from build123d import *

# Parameters (mm, degrees)
BOX042_W                  = 13
BOX042_H                  = 42
BOX042_DEPTH              = 6
BOX043_W                  = 9
BOX043_H                  = 58
BOX043_DEPTH              = 2
CYLINDER024_R             = 20.5
CYLINDER024_DEPTH         = 23.5
FUSION001_PITCH_ANGLE     = -90
FUSION001_PLACEMENT_ANGLE = 90


with BuildPart() as cube022:
    # Box042 → Box042 (new body)
    with BuildSketch(Plane(origin=(-6.5, -21, 0), x_dir=(1, 0, 0), z_dir=(0, 0, 1))):
        with Locations((6.5, 21)):
            Rectangle(BOX042_W, BOX042_H)
    extrude(amount=BOX042_DEPTH)


with BuildPart() as cube023:
    # Box043 → Box043 (new body)
    with BuildSketch(Plane(origin=(-4.5, -29, 5.5), x_dir=(1, 0, 0), z_dir=(0, 0, 1))):
        with Locations((4.5, 29)):
            Rectangle(BOX043_W, BOX043_H)
    extrude(amount=BOX043_DEPTH)


with BuildPart() as speaker:
    # Cylinder024 → Cylinder024 (new body)
    with BuildSketch(Plane.XY):
        Circle(CYLINDER024_R)
    extrude(amount=CYLINDER024_DEPTH)

    # Fusion001: union Cube022, Cube023
    add(cube022.part)
    add(cube023.part)


with BuildPart() as speaker_1:
    # Fusion001 pitch: moved
    add(speaker.part.rotate(Axis((0, 0, 0), (0, 1, 0)), FUSION001_PITCH_ANGLE))


with BuildPart() as speaker_2:
    # Fusion001 placement: moved
    add(speaker_1.part.moved(Location((45, 86, 45))).rotate(Axis((45, 86, 45), (0, 0, 1)), FUSION001_PLACEMENT_ANGLE))


solid = speaker_2.part
Geometry: final body of the model. Coordinates: model frame, mm. A direction names the side the tool comes from. Round coordinates to 2 decimals unless told otherwise and drop trailing zeros. Write each loop counter-clockwise with the first axis right and the second up, starting at its lowest first coordinate (ties: lowest second). Pieces come first, ordered by that corner, then holes. Notation, with made-up numbers: M 84,-22 L 130,-22 A10 ccw 130,-13 Z; hole C 20,3.25 d1. An arc over 180 degrees is marked long. Write item = value, one per line.
Item 1: Material intervals for line 1 along X through (y, z) = (74.25, 38.5); line 2 along Y through (x, z) = (20.5, 41); line 3 along X through (y, z) = (66.5, 42.5), sorted ascending. Write a range as [from, to].
Findings:
line_1 = [25.56, 64.44]
line_2 = [78.5, 80.5]
line_3 = [24.65, 65.35]
Item 2: Section query A-A on y = 83.5. Return loops of the section in (x, z), then the cut area to 3 significant figures.
Findings:
outline = M 24,38.5 L 25.56,38.5 A20.5 ccw 64.44,38.5 L 66,38.5 L 66,51.5 L 64.44,51.5 A20.5 ccw 25.56,51.5 L 24,51.5 Z
area = 1,340 mm^2
Item 3: Access query for faces 1 (the face through (65, 80, 39)), 2 (the face through (20, 80.5, 45)), 3 (the face through (65, 83, 51.5)). Directions: +Z, -Z, +X, -X, +Y, -Y. A direction counts if a zero-diameter tool reaches every point of the face in a straight line with its end or side. Return the directions, or none.
Findings:
face_1 = -Z, +X, -Y
face_2 = +Z, -Z, -X, +Y
face_3 = +Z, +X, +Y, -Y
Item 4: Section query B-B on z = 45. Return loops of the section in (x, y).
Findings:
outline = M 16,78.5 L 24.5,78.5 L 24.5,62.5 L 65.5,62.5 L 65.5,78.5 L 74,78.5 L 74,80.5 L 66,80.5 L 66,86 L 24,86 L 24,80.5 L 16,80.5 Z
Item 5: Section query C-C on x = 70. Return loops of the section in (y, z), then the cut area to 3 significant figures.
Findings:
outline = M 78.5,40.5 L 80.5,40.5 L 80.5,49.5 L 78.5,49.5 Z
area = 18.0 mm^2
Item 6: Section query D-D on y = 74.25. Return loops of the section in (x, z), then the cut area to 3 significant figures.
Findings:
outline = C 45,45 d41
area = 1,320 mm^2
Item 7: Pin query (flat end, axial travel): P1, Ø1, axis at x = 70, y = 79, coming from the +Z side; P2, Ø6.5, axis at y = 84, z = 45, coming from the -X side; P3, Ø3, axis at y = 82, z = 54, coming from the -X side. Return the tip coordinate at first contact, or that it passes through.
Findings:
P1 = 49.5
P2 = 24
P3 = 25.92
